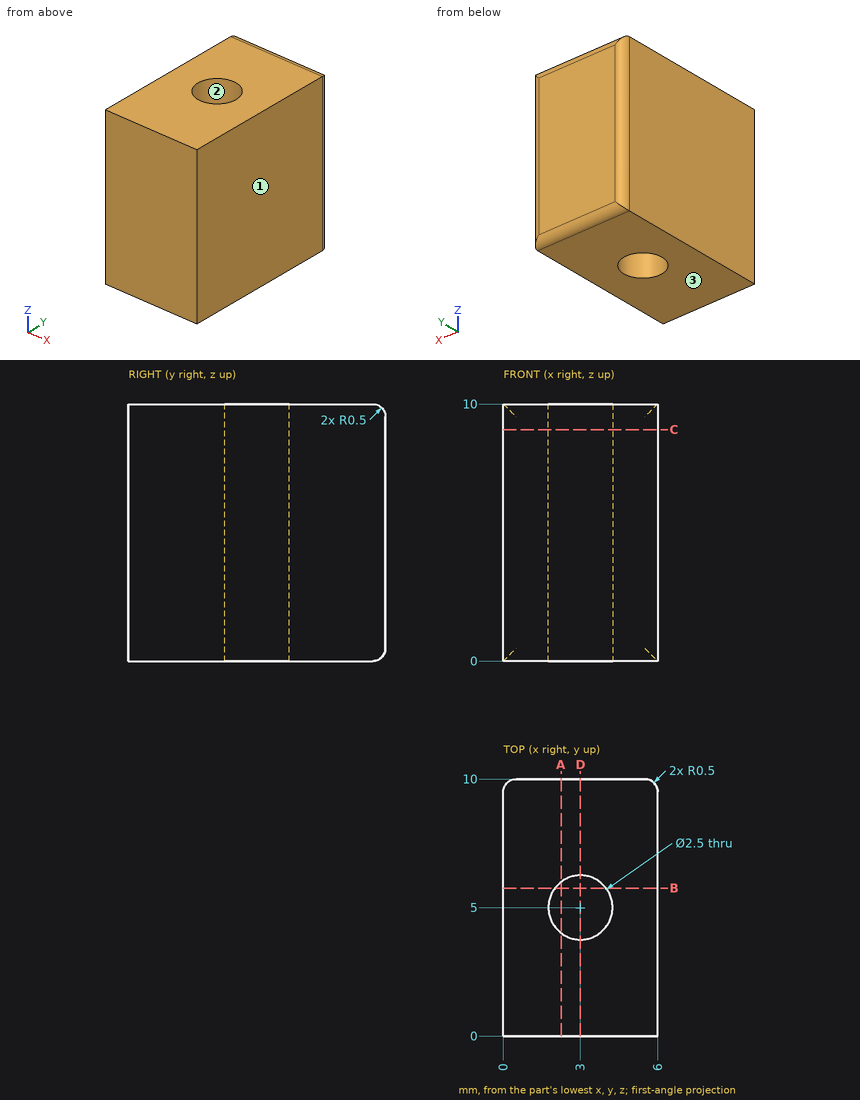
Input: dimensioned drawing with shaded views. Units: mm. Origin: part minimum x, y, z. Coordinates: 2 decimals unless noted, no trailing zeros. Loops run counter-clockwise (first coordinate to the right, second up) from the corner with the lowest first, then second, coordinate; pieces in that order, holes last. Notation, with made-up numbers: M 30,-37 L 34,-37 A29 ccw 34,-14 Z; hole C 29,-14.5 d3. An arc over 180 degrees is marked long. Use a Markdown table: item, result. Add a question column.
Q1. Section query D-D, the plane x = 3. Return loops of the section in (y, z), and give its area (3 significant figures).
Q2. Material intervals for L1, parallel to Y at x = 3, z = 4.25; L2, parallel to X at y = 4.5, z = 8; L3, parallel to Y at x = 5.75, z = 3, sorted ascending.
Q3. Section query B-B, the plane y = 5.75. Return loops of the section in (x, z).
Q4. Section query C-C, the plane z = 9. Return loops of the section in (x, y).
Q5. Section query A-A, the plane x = 2.25. Return loops of the section in (y, z).
Q6. Draft query along X for the marked faces 1, 2 and 3. Return one class per face: pulls with the +X half, pulls with the -X half, needs draft (parallel to the pull), parting line crosses it, or undercut.
Result:
| question | item | result |
|---|---|---|
| 1 | outline | M 0,0 L 3.75,0 L 3.75,10 L 0,10 Z; M 6.25,0 L 9.5,0 A0.5 ccw 10,0.5 L 10,9.5 A0.5 ccw 9.5,10 L 6.25,10 Z |
| 1 | area | 74.9 mm2 |
| 2 | L1 | y = 0 to 3.75, 6.25 to 10 |
| 2 | L2 | x = 0 to 1.85, 4.15 to 6 |
| 2 | L3 | y = 0 to 9.93 |
| 3 | outline | M 0,0 L 2,0 L 2,10 L 0,10 Z; M 4,0 L 6,0 L 6,10 L 4,10 Z |
| 4 | outline | M 0,0 L 6,0 L 6,9.5 A0.5 ccw 5.5,10 L 0.5,10 A0.5 ccw 0,9.5 Z; hole C 3,5 d2.5 |
| 5 | outline | M 0,0 L 4,0 L 4,10 L 0,10 Z; M 6,0 L 9.5,0 A0.5 ccw 10,0.5 L 10,9.5 A0.5 ccw 9.5,10 L 6,10 Z |
| 6 | face 1 | pulls with the +X half |
| 6 | face 2 | undercut |
| 6 | face 3 | needs draft |
